from build123d import *

# Parameters (mm, degrees)
SKETCH_1_R          = 5
EXTRUDE_1_DEPTH     = 12
SKETCH_2_R          = 2.5
CUT_EXTRUDE_1_DEPTH = 10


with BuildPart() as part:
    # 草图1 → 凸台-拉伸1 (new body)
    with BuildSketch(Plane.XY):
        with BuildLine():
            Line((12.5, 0), (12.5, -29.5))
            ThreePointArc((12.5, -29.5), (10.021323251, -32.847670655), (6.096057819, -31.453745072))
            Line((6.096057819, -31.453745072), (-10.371222076, -6.977660972))
            Line((-10.371222076, -6.977660972), (-27.427039052, 18.373193167))
            ThreePointArc((-27.427039052, 18.373193167), (-32.822608292, 23.240050935), (-39.872505543, 25))
            Line((-39.872505543, 25), (-45, 25))
            ThreePointArc((-45, 25), (-46.767766953, 25.732233047), (-47.5, 27.5))
            Line((-47.5, 27.5), (-47.5, 37.5))
            ThreePointArc((-47.5, 37.5), (-46.767766953, 39.267766953), (-45, 40))
            Line((-45, 40), (30, 40))
            ThreePointArc((30, 40), (31.767766953, 39.267766953), (32.5, 37.5))
            Line((32.5, 37.5), (32.5, 27.5))
            ThreePointArc((32.5, 27.5), (31.767766953, 25.732233047), (30, 25))
            Line((30, 25), (27.5, 25))
            ThreePointArc((27.5, 25), (16.893398282, 20.606601718), (12.5, 10))
            Line((12.5, 10), (12.5, 0))
        make_face()
        Circle(SKETCH_1_R, mode=Mode.SUBTRACT)
    extrude(amount=EXTRUDE_1_DEPTH)

    # 草图2 → 切除-拉伸1 (cut)
    with BuildSketch(Plane(origin=(0, 40, 0), x_dir=(1, 0, 0), z_dir=(0, 1, 0))):
        with Locations(Location((-30, -6, 0), (0, 0, 270))):
            Circle(SKETCH_2_R)
        with Locations(Location((-15, -6, 0), (0, 0, 270))):
            Circle(SKETCH_2_R)
        with Locations(Location((0, -6, 0), (0, 0, 270))):
            Circle(SKETCH_2_R)
        with Locations(Location((15, -6, 0), (0, 0, 270))):
            Circle(SKETCH_2_R)
    extrude(amount=-CUT_EXTRUDE_1_DEPTH, mode=Mode.SUBTRACT)


solid = part.part
Design review of the part built by this model. Coordinates are the model's own, in mm. A direction names the side the tool comes from. Round coordinates to 2 decimals unless told otherwise and drop trailing zeros. Write each loop counter-clockwise with the first axis right and the second up, starting at its lowest first coordinate (ties: lowest second). Pieces come first, ordered by that corner, then holes. Notation, with made-up numbers: (70, -30.5) - (81, -30.5) arc R24 ccw to (81, 2.5) - close; hole circle Ø6 at (15.25, 46). An arc over 180 degrees is marked (long way). Use a Markdown table: item, result. Add a question column.
1. For faces 4 (the face through (-30, 30, 6)), 5 (the face through (12.5, -9, 6)), 6 (the face through (-47.5, 32, 6)), list the 3-axis set-ups (+Z, -Z, +X, -X, +Y, -Y) from which the entire face can be reached by the end or side of a thin tool; tool diameter is ignored.
2. Mouldability with a two-part tool opening along Z and no side actions: class faces 1 (the face through (0.751, 35.07, 8.385)), 2 (the face through (-8, 40, 6)), 3 (the face through (-7, 20, 12)) as +Z half, -Z half, draft (parallel to the pull), parting line (faces both ways), or undercut.
3. Wall thickness on probe 1 along X at (y, z) = (34.5, 6); probe 2 along X at (y, z) = (38.25, 6); probe 3 along Y at (x, z) = (3.5, 2.75): over which ranges is each line inside the solid? List them lowest first.
4. We need section D-D (x = -31). State the section outline as (y, z) points, then the cut area to 3 significant figures.
5. Clearance check with flat-ended pins moving along their axes: pin 1 (5 mm diameter, centred on x = -34, z = 9.5, fed in from -Y); pin 2 (0.8 mm diameter, centred on x = 28.5, z = 7.5, fed in from -Y); pin 3 (4 mm diameter, centred on x = 0, z = 6, fed in from +Y). State where each tip first meets the part, or that it passes through.
6. We need section B-B (x = 0). State the section outline as (y, z) points, then the cut area to 3 significant figures.
7. We need section C-C (y = 0). State the section outline as (x, z) points, then the cut area to 3 significant figures.
Output:
| question | item | result |
|---|---|---|
| 1 | face 4 | +Y |
| 1 | face 5 | +Z, -Z, +X, -Y |
| 1 | face 6 | +Z, -Z, -X, +Y, -Y |
| 2 | face 1 | undercut |
| 2 | face 2 | draft |
| 2 | face 3 | +Z half |
| 3 | probe 1 | x = -47.5 to -32.5, -27.5 to -17.5, -12.5 to -2.5, 2.5 to 12.5, 17.5 to 32.5 |
| 3 | probe 2 | x = -47.38 to -32.5, -27.5 to -17.5, -12.5 to -2.5, 2.5 to 12.5, 17.5 to 32.38 |
| 3 | probe 3 | y = -27.6 to -3.57, 3.57 to 40 |
| 4 | outline | (22.09, 0) - (40, 0) - (40, 3.71) - (30, 3.71) - (30, 8.29) - (40, 8.29) - (40, 12) - (22.09, 12) - close |
| 4 | area | 169 mm2 |
| 5 | pin 1 | stops at y = 22.45 |
| 5 | pin 2 | stops at y = 25 |
| 5 | pin 3 | stops at y = 30 |
| 6 | outline | (-22.39, 0) - (-5, 0) - (-5, 12) - (-22.39, 12) - close; (5, 0) - (40, 0) - (40, 3.5) - (30, 3.5) - (30, 8.5) - (40, 8.5) - (40, 12) - (5, 12) - close |
| 6 | area | 579 mm2 |
| 7 | outline | (-15.07, 0) - (-5, 0) - (-5, 12) - (-15.07, 12) - close; (5, 0) - (12.5, 0) - (12.5, 12) - (5, 12) - close |
| 7 | area | 211 mm2 |
